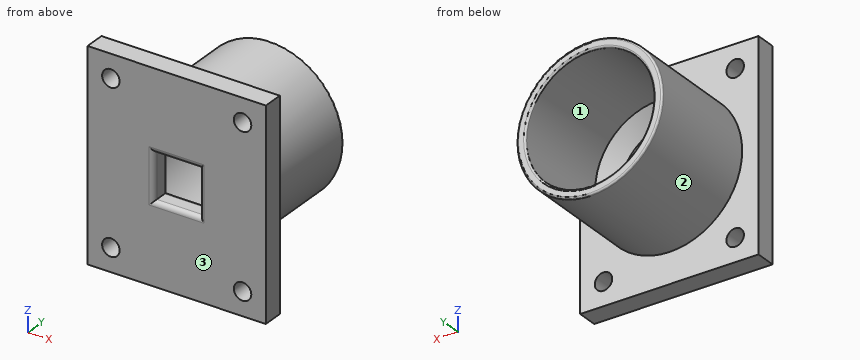
Autodesk Inventor part; units mm, degrees
ref_plane "YZ Plane" through (0, 0, 0) normal (1, 0, 0) x (0, 1, 0)
ref_plane "XZ Plane" through (0, 0, 0) normal (0, 1, 0) x (-1, 0, 0)
ref_plane "XY Plane" through (0, 0, 0) normal (0, 0, 1) x (1, 0, 0)
sketch "Sketch1" plane through (0, 0, 0) normal (0, 1, 0) x (-1, 0, 0)
  line L0 (19.431, 22.5) -> (-19.431, 22.5)
  line L1 (-19.431, 22.5) -> (-19.431, -22.5)
  line L2 (-19.431, -22.5) -> (19.431, -22.5)
  line L3 (19.431, -22.5) -> (19.431, 22.5)
  line L4 (19.431, 22.5) -> (-19.431, -22.5) construction
  line L5 (-19.431, 22.5) -> (19.431, -22.5) construction
  point P0 (0, 0)
  dimension "d0" = 38.862
  dimension "d1" = 45
extrude "ExtrusionForFloor" add sketch "Sketch1" against normal blind 4.445
sketch "Sketch4" plane through (0, 0, 0) normal (0, 1, 0) x (1, 0, 0)
  line L0 (-5, -5) -> (5, -5)
  line L1 (5, -5) -> (5, 5)
  line L2 (5, 5) -> (-5, 5)
  line L3 (-5, 5) -> (-5, -5)
  line L4 (-5, -5) -> (5, 5) construction
  line L5 (5, -5) -> (-5, 5) construction
  point P0 (0, 0)
  dimension "d21" = 10
extrude "ExtrusionForCameraHole" cut sketch "Sketch4" against normal through all
sketch "Sketch5" plane through (0, -4.445, 0) normal (0, -1, 0) x (1, 0, 0)
  line L0 (18.161, 21.23) -> (-18.161, 21.23)
  line L1 (-18.161, 21.23) -> (-18.161, -21.23)
  line L2 (-18.161, -21.23) -> (18.161, -21.23)
  line L3 (18.161, -21.23) -> (18.161, 21.23)
  line L4 (18.161, 21.23) -> (-18.161, -21.23) construction
  line L5 (-18.161, 21.23) -> (18.161, -21.23) construction
  line L6 (19.431, -22.5) -> (19.431, 22.5)
  line L7 (19.431, 22.5) -> (-19.431, 22.5)
  line L8 (19.431, 22.5) -> (-19.431, 22.5)
  line L9 (-19.431, 22.5) -> (-19.431, -22.5)
  line L10 (-19.431, -22.5) -> (19.431, -22.5)
  line L11 (19.431, -22.5) -> (19.431, 22.5)
  line L12 (-19.431, 22.5) -> (-19.431, -22.5)
  line L13 (-19.431, -22.5) -> (19.431, -22.5)
  point P0 (0, 0)
  dimension "d24" = 1.27
  dimension "d25" = 1.27
  dimension "d41" = 0
  dimension "d43" = 0
sketch "Sketch7" plane through (0, 0, 0) normal (0, 1, 0) x (1, 0, 0)
  circle A0 centre (0, 0) radius 15.875
  circle A1 centre (0, 0) radius 13.97
  dimension "d32" = 31.75
  dimension "d33" = 27.94
extrude "ExtrusionForEyepieceAttachement" add sketch "Sketch7" along normal blind 25.4
sketch "Sketch19" plane through (0, 0, 0) normal (0, 1, 0) x (1, 0, 0)
  circle A0 centre (-14.351, 17.42) radius 1.2192
  circle A1 centre (-14.351, -17.42) radius 1.2192
  circle A2 centre (14.351, -17.42) radius 1.2192
  circle A3 centre (14.351, 17.42) radius 1.2192
  line L0 (19.431, -22.5) -> (19.431, 22.5)
  line L1 (-19.431, 22.5) -> (-19.431, -22.5)
  line L2 (-19.431, -22.5) -> (19.431, -22.5)
  line L3 (19.431, 22.5) -> (-19.431, 22.5)
  point P0 (0, 0)
  dimension "d104" = 5.08
  dimension "d105" = 5.08
  dimension "d106" = 5.08
  dimension "d107" = 5.08
  dimension "d108" = 5.08
  dimension "d109" = 5.08
  dimension "d110" = 5.08
  dimension "d111" = 5.08
hole "Hole5" at (-14.351, 0, -17.42) at (-14.351, 0, 17.42) at (14.351, 0, 17.42) at (14.351, 0, -17.42) direction (0, -1, 0) diameter 3.81 end through all
fillet "Fillet3" radius 0.3969 2 edges at (-15.875, 25.4, 0) (-13.97, 25.4, 0)
fillet "Fillet4" radius 1 4 edges at (-5, -4.445, 0) (0, -4.445, -5) (5, -4.445, 0) (0, -4.445, 5)
fillet "Fillet5" radius 1 4 edges at (0, 0, 5) (-5, 0, 0) (0, 0, -5) (5, 0, 0)
chamfer "Chamfer2" distance 3.175 angle 45 1 edges at (-13.97, 0, 0)
equation "\"d1\" = CaseWidth"
equation "\"d21\" = PiCameraLensCover"
equation "\"d24\" = CaseWallThickness"
equation "\"d25\" = CaseWallThickness"
equation "\"d32\" = EyepieceOutsideDiameter"
equation "\"d33\" = EyepieceInnerDiameter"
equation "\"d34\" = EyepieceAdapterLength"
equation "\"PiCameraLength\" = 23.862"
equation "\"PiCameraWidth\" = 25"
equation "\"PiCameraLensCover\" = 10"
equation "\"EyepieceAdapterLength\" = 25.4"
equation "\"OffsetForBoltPattern\" = 3.175"
equation "\"FloorThickness\" = 1.905"
equation "\"SlotForEyepiece\" = 2.54"
properties part number "TelescopeAttachementForCase" material "Polypropylene"
Work out the finished part from the listing and answer in its coordinate system (mm). Face numbers are marked on the shaded views. Coordinates: 2 decimals unless noted, no trailing zeros. Loops run counter-clockwise (first coordinate to the right, second up) from the corner with the lowest first, then second, coordinate; pieces in that order, holes last. Notation, with made-up numbers: (17, 3) -> (72, 3) arc R20 cw to (72, 16) -> close; hole circle Ø7 at (-11.75, -0.75). An arc over 180 degrees is marked (long way). Answer as CSV lines item,"result".
Q1. The part is cut by section A-A on z = -17.42. Write down the section's boundary in (x, y) (3 decimals), and give its area (3 significant figures).
Findings:
outline,"(-19.431, -4.445) -> (-16.256, -4.445) -> (-16.256, 0) -> (-19.431, 0) -> close; (-12.446, -4.445) -> (12.446, -4.445) -> (12.446, 0) -> (-12.446, 0) -> close; (16.256, -4.445) -> (19.431, -4.445) -> (19.431, 0) -> (16.256, 0) -> close"
area,"139 mm²"
Q2. Each of these flat-tipped pins is pushed along its axis until it touches: pin 1 (6.5 mm diameter, centred on x = -4, z = 2, fed in from +Y); pin 2 (10 mm diameter, centred on x = -2, y = 17.5, fed in from +Z) (3 decimals); pin 3 (3.5 mm diameter, centred on x = 14.351, z = -17.42, fed in from -Y); pin 4 (10 mm diameter, centred on x = -10.5, z = 5.5, fed in from +Y). Where does it stop, or does it pass through?
Findings:
pin 1,"stops at y = 0"
pin 2,"stops at z = 15.875"
pin 3,"passes through"
pin 4,"stops at y = 25.4"
Q3. The part is cut by section B-B on x = 0. Write down the section's boundary in (y, z) (3 decimals).
Findings:
outline,"(-4.445, -22.5) -> (0, -22.5) -> (0, -15.875) -> (25.003, -15.875) arc R0.397 ccw to (25.4, -15.478) -> (25.4, -14.367) arc R0.397 ccw to (25.003, -13.97) -> (3.175, -13.97) -> (0, -10.795) -> (0, -6) arc R1 ccw to (-1, -5) -> (-3.445, -5) arc R1 ccw to (-4.445, -6) -> close; (-4.445, 6) arc R1 ccw to (-3.445, 5) -> (-1, 5) arc R1 ccw to (0, 6) -> (0, 10.795) -> (3.175, 13.97) -> (25.003, 13.97) arc R0.397 ccw to (25.4, 14.367) -> (25.4, 15.478) arc R0.397 ccw to (25.003, 15.875) -> (0, 15.875) -> (0, 22.5) -> (-4.445, 22.5) -> close"
Q4. The part is cut by section C-C on z = 0. Write down the section's boundary in (x, y) (3 decimals).
Findings:
outline,"(-19.431, -4.445) -> (-6, -4.445) arc R1 ccw to (-5, -3.445) -> (-5, -1) arc R1 ccw to (-6, 0) -> (-10.795, 0) -> (-13.97, 3.175) -> (-13.97, 25.003) arc R0.397 ccw to (-14.367, 25.4) -> (-15.478, 25.4) arc R0.397 ccw to (-15.875, 25.003) -> (-15.875, 0) -> (-19.431, 0) -> close; (5, -3.445) arc R1 ccw to (6, -4.445) -> (19.431, -4.445) -> (19.431, 0) -> (15.875, 0) -> (15.875, 25.003) arc R0.397 ccw to (15.478, 25.4) -> (14.367, 25.4) arc R0.397 ccw to (13.97, 25.003) -> (13.97, 3.175) -> (10.795, 0) -> (6, 0) arc R1 ccw to (5, -1) -> close"
Q5. Find the intervals of material crossed by probe 1 along X at (y, z) = (-2.9, 17.42); probe 2 along X at (y, z) = (18, 0) (3 decimals); probe 3 along Z at (x, y) = (16, -1.25), in increasing order.
Findings:
probe 1,"x = -19.43 to -16.26, -12.45 to 12.45, 16.26 to 19.43"
probe 2,"x = -15.875 to -13.97, 13.97 to 15.875"
probe 3,"z = -22.5 to -18.37, -16.47 to 16.47, 18.37 to 22.5"
Q6. The part is cut by section D-D on y = 15. Write down the section's boundary in (x, z) (3 decimals).
Findings:
outline,"circle Ø31.75 at (0, 0); hole circle Ø27.94 at (0, 0)"
Q7. For a pull along Z with two mould halves and no side action, classify the marked faces 1, 2 and 3 as +Z half, -Z half, draft (parallel to the pull), parting line (faces both ways), or undercut.
Findings:
face 1,"undercut"
face 2,"parting line"
face 3,"draft"
